from build123d import *

# Parameters (mm, degrees)
BOSS_EXTRUDE1_DEPTH = 42
CUT_EXTRUDE1_REACH  = 14.828
SKETCH2_R           = 1.5
CUT_EXTRUDE2_REACH  = 6
SKETCH3_R           = 1.5
SKETCH3_R_2         = 19
CUT_EXTRUDE3_DEPTH  = 4
CUT_EXTRUDE4_DEPTH  = 4


with BuildPart() as part:
    # Sketch1 → Boss-Extrude1 (new body)
    with BuildSketch(Plane(origin=(0, 0, 0), x_dir=(1, 0, 0), z_dir=(0, 1, 0))):
        Polygon((0, 0), (51.656854249, 0), (51.656854249, -4), (1.656854249, -4), (-9.656854249, -15.313708499), (-12.485281374, -12.485281374), align=None)
    extrude(amount=BOSS_EXTRUDE1_DEPTH)

    # Sketch2 → Cut-Extrude1 (cut, up to next)
    with BuildSketch(Plane(origin=(2.828427125, 0, 2.828427125), x_dir=(0.707106781, 0, -0.707106781), z_dir=(0.707106781, 0, 0.707106781)), mode=Mode.PRIVATE) as cut_extrude1_sk1:
        with Locations((-14.656854249, 34)):
            Circle(SKETCH2_R)
    cut_extrude1_tool1 = extrude(cut_extrude1_sk1.sketch, amount=-CUT_EXTRUDE1_REACH, mode=Mode.PRIVATE) & part.part
    add(cut_extrude1_tool1.solids().sort_by_distance((-7.535534, 34, 13.192388))[0], mode=Mode.SUBTRACT)
    # Sketch2 → Cut-Extrude1 (cut, up to next)
    with BuildSketch(Plane(origin=(2.828427125, 0, 2.828427125), x_dir=(0.707106781, 0, -0.707106781), z_dir=(0.707106781, 0, 0.707106781)), mode=Mode.PRIVATE) as cut_extrude1_sk2:
        with Locations((-14.656854249, 8)):
            Circle(SKETCH2_R)
    cut_extrude1_tool2 = extrude(cut_extrude1_sk2.sketch, amount=-CUT_EXTRUDE1_REACH, mode=Mode.PRIVATE) & part.part
    add(cut_extrude1_tool2.solids().sort_by_distance((-7.535534, 8, 13.192388))[0], mode=Mode.SUBTRACT)

    # Sketch3 → Cut-Extrude2 (cut, up to next)
    with BuildSketch(Plane.XY.offset(4), mode=Mode.PRIVATE) as cut_extrude2_sk1:
        with Locations((14.656854249, 37)):
            Circle(SKETCH3_R)
    cut_extrude2_tool1 = extrude(cut_extrude2_sk1.sketch, amount=-CUT_EXTRUDE2_REACH, mode=Mode.PRIVATE) & part.part
    add(cut_extrude2_tool1.solids().sort_by_distance((14.656854, 37, 4))[0], mode=Mode.SUBTRACT)
    # Sketch3 → Cut-Extrude2 (cut, up to next)
    with BuildSketch(Plane.XY.offset(4), mode=Mode.PRIVATE) as cut_extrude2_sk2:
        with Locations((46.656854249, 37)):
            Circle(SKETCH3_R)
    cut_extrude2_tool2 = extrude(cut_extrude2_sk2.sketch, amount=-CUT_EXTRUDE2_REACH, mode=Mode.PRIVATE) & part.part
    add(cut_extrude2_tool2.solids().sort_by_distance((46.656854, 37, 4))[0], mode=Mode.SUBTRACT)
    # Sketch3 → Cut-Extrude2 (cut, up to next)
    with BuildSketch(Plane.XY.offset(4), mode=Mode.PRIVATE) as cut_extrude2_sk3:
        with Locations((46.656854249, 5)):
            Circle(SKETCH3_R)
    cut_extrude2_tool3 = extrude(cut_extrude2_sk3.sketch, amount=-CUT_EXTRUDE2_REACH, mode=Mode.PRIVATE) & part.part
    add(cut_extrude2_tool3.solids().sort_by_distance((46.656854, 5, 4))[0], mode=Mode.SUBTRACT)
    # Sketch3 → Cut-Extrude2 (cut, up to next)
    with BuildSketch(Plane.XY.offset(4), mode=Mode.PRIVATE) as cut_extrude2_sk4:
        with Locations((14.656854249, 5)):
            Circle(SKETCH3_R)
    cut_extrude2_tool4 = extrude(cut_extrude2_sk4.sketch, amount=-CUT_EXTRUDE2_REACH, mode=Mode.PRIVATE) & part.part
    add(cut_extrude2_tool4.solids().sort_by_distance((14.656854, 5, 4))[0], mode=Mode.SUBTRACT)
    # Sketch3 → Cut-Extrude2 (cut, up to next)
    with BuildSketch(Plane.XY.offset(4), mode=Mode.PRIVATE) as cut_extrude2_sk5:
        with Locations((30.656854249, 21)):
            Circle(SKETCH3_R_2)
    cut_extrude2_tool5 = extrude(cut_extrude2_sk5.sketch, amount=-CUT_EXTRUDE2_REACH, mode=Mode.PRIVATE) & part.part
    add(cut_extrude2_tool5.solids().sort_by_distance((30.656854, 21, 4))[0], mode=Mode.SUBTRACT)

    # Sketch6 → Cut-Extrude3 (cut)
    with BuildSketch(Plane(origin=(0, 0, 0), x_dir=(-0.707106781, 0, 0.707106781), z_dir=(-0.707106781, 0, -0.707106781))):
        with BuildLine():
            Line((0, 5), (0, 0))
            Line((0, 0), (11.180339887, 0))
            ThreePointArc((11.180339887, 0), (6.123724357, 3.693063938), (0, 5))
        make_face()
        with BuildLine():
            Line((0, 37), (0, 42))
            Line((0, 42), (11.180339887, 42))
            ThreePointArc((11.180339887, 42), (6.123724357, 38.306936062), (0, 37))
        make_face()
    extrude(amount=-CUT_EXTRUDE3_DEPTH, mode=Mode.SUBTRACT)

    # Sketch7 → Cut-Extrude4 (cut)
    with BuildSketch(Plane(origin=(0, 0, 0), x_dir=(-1, 0, 0), z_dir=(0, 0, -1))):
        with BuildLine():
            Line((-9.746794345, 42), (0, 42))
            Line((0, 42), (0, 37))
            ThreePointArc((0, 37), (-5.477225575, 38.322921748), (-9.746794345, 42))
        make_face()
        with BuildLine():
            Line((-9.746794345, 0), (0, 0))
            Line((0, 0), (0, 5))
            ThreePointArc((0, 5), (-5.477225575, 3.677078252), (-9.746794345, 0))
        make_face()
    extrude(amount=-CUT_EXTRUDE4_DEPTH, mode=Mode.SUBTRACT)


solid = part.part
Read the model definition and answer for the solid it produces. Units are mm, in the model's axes. A direction names the side the tool comes from. Round coordinates to 2 decimals unless told otherwise and drop trailing zeros. Order: outer loops, then holes, each group sorted by start corner. A loop starts at its lowest first (then second) coordinate and runs counter-clockwise, first axis right, second up.
1) The part is cut by section D-D on x = 24. Write down the section's boundary in (y, z), plus the area to 3 significant figures.
2) Straight lines are drawn through the part: L1, parallel to Y at x = -9, z = 11.5; L2, parallel to X at y = 6, z = 3; L3, parallel to Z at x = 17.5, y = 5. For each, find the intervals that lie inside material, in ascending order.
3) The part is cut by section C-C on y = 26. Write down the section's boundary in (x, z).
4) The part is cut by section A-A on y = 21. Write down the section's boundary in (x, z).
5) The part is cut by section B-B on x = 35. Write down the section's boundary in (y, z).
6) The mould has two halves that part along Z. Classify faces 3 (the face through (-9.16, 32.536, 12.028)), 4 (the face through (-3.921, 20.706, 9.578)), 5 (the face through (31, 0, 2)): released by +Z, released by -Z, zero draft, split by the parting line, or undercut.
7) For faces 1 (the face through (16.088, 5.451, 2.028)), 2 (the face through (0.421, 4.993, 2.861)), determine the directions among +Z, -Z, +X, -X, +Y, -Y from which every point of the face is accessible in a straight line to the end or side of a thin tool.
8) Flat-ended cylindrical pins translate along their axes: pin 1 (5 mm diameter, centred on y = 24, z = 3, fed in from -X); pin 2 (8 mm diameter, centred on y = 9.5, z = 11, fed in from +X); pin 3 (4 mm diameter, centred on x = 46.66, y = 37, fed in from +Z). Find the tip coordinate at first contact, or state that the pin passes through.
Resolved:
1. outline: (0, 0) - (3.2, 0) - (3.2, 4) - (0, 4) - close; (38.8, 0) - (42, 0) - (42, 4) - (38.8, 4) - close
1. area: 25.6 mm2
2. L1: y = 0 to 6.51, 9.49 to 32.51, 35.49 to 42
2. L2: x = -3 to 13.54, 15.77 to 18.99, 42.32 to 45.54, 47.77 to 51.66
2. L3: z = 0 to 4
3. outline: (-12.49, 12.49) - (0, 0) - (12.33, 0) - (12.33, 4) - (1.66, 4) - (-9.66, 15.31) - close; (48.99, 0) - (51.66, 0) - (51.66, 4) - (48.99, 4) - close
4. outline: (-12.49, 12.49) - (0, 0) - (11.66, 0) - (11.66, 4) - (1.66, 4) - (-9.66, 15.31) - close; (49.66, 0) - (51.66, 0) - (51.66, 4) - (49.66, 4) - close
5. outline: (0, 0) - (2.5, 0) - (2.5, 4) - (0, 4) - close; (39.5, 0) - (42, 0) - (42, 4) - (39.5, 4) - close
6. face 3: undercut
6. face 4: released by +Z
6. face 5: zero draft
7. face 1: +Z, -Z
7. face 2: -Z, -Y
8. pin 1: stops at x = -5.5
8. pin 2: stops at x = -1.34
8. pin 3: stops at z = 4
